Check sheet for the modelled part. Datum: model origin and axes. Units: mm. A direction names the side the tool comes from. Give positions to 0.01 mm unless a question says otherwise; leave off trailing zeros. Write each loop counter-clockwise with the first axis right and the second up, starting at its lowest first coordinate (ties: lowest second). Pieces come first, ordered by that corner, then holes. Notation, with made-up numbers: M -21.75,-32 L 26.25,-32 A22 cw 26.25,-25 Z; hole C 78.5,53 d10. An arc over 180 degrees is marked long. Write item = value, one per line. Start each with the question number.
1) Cross-section at A-A, the plane x = 13. Record the cut outline in (y, z) (3 decimals).
2) Access from +Z, -Z, +X, -X, +Y, -Y to the whole of each face (thin tool, end or side, straight path). Record for faces 4 (the cylindrical face through (0.456, 50.245, 136.744)), 5 (the flat face through (0, 25, 0)).
3) Mould release check, pull along Z, two halves, no side actions. Record for faces 1 (the cylindrical face through (0.46, 50.21, 23.34)), 2 (the flat face through (0, 25, 152.4)), 3 (the flat face through (-14.989, 19, 75)): released by +Z, released by -Z, zero draft, split by the parting line, or undercut.
4) Go/stop test with a flat-tipped pin: pin 1 (8 mm diameter, centred on x = -8, z = 66.5, fed in from +Y). Record where the tip stops, or that it passes through.
5) Scan lines: line 1 along Y through (x, z) = (1.5, 79.5); line 2 along Y through (x, z) = (14, 101); line 3 along Z through (x, y) = (-9.5, 48). Record each from-to range of solid material in increasing order. Write a range as [from, to].
```python
from build123d import *

# Parameters (mm, degrees)
F0_W     = 30.48
F0_H     = 152.4
F1_DEPTH = 50.8
F3_DEPTH = 30.481
F4_R     = 5.08


with BuildPart() as f1:
    # F0 (on Front) → F1 (new body)
    with BuildSketch(Plane.XZ):
        with Locations((0.2509840885, 76.2)):
            Rectangle(F0_W, F0_H)
    extrude(amount=-F1_DEPTH)

    # F2 (on face) → F3 (cut, through all)
    with BuildSketch(Plane.YZ.offset(15.4909840885)):
        with BuildLine():
            ThreePointArc((65.3252072253, 107.95), (71.4179823352, 113.7862789789), (73.66, 121.92))
            ThreePointArc((73.66, 121.92), (49.6512789789, 135.5529823352), (50.2447927747, 107.95))
            ThreePointArc((50.2447927747, 107.95), (57.785, 109.855), (65.3252072253, 107.95))
        make_face()
        with BuildLine():
            ThreePointArc((65.3252072253, 107.95), (57.785, 109.855), (50.2447927747, 107.95))
            ThreePointArc((50.2447927747, 107.95), (57.785, 106.045), (65.3252072253, 107.95))
        make_face()
        with BuildLine():
            ThreePointArc((65.3252072253, 107.95), (57.785, 106.045), (50.2447927747, 107.95))
            ThreePointArc((50.2447927747, 107.95), (41.91, 93.98), (50.2447927747, 80.01))
            ThreePointArc((50.2447927747, 80.01), (57.785, 81.915), (65.3252072253, 80.01))
            ThreePointArc((65.3252072253, 80.01), (71.4179823352, 85.8462789789), (73.66, 93.98))
            ThreePointArc((73.66, 93.98), (71.4179823352, 102.1137210211), (65.3252072253, 107.95))
        make_face()
        with BuildLine():
            ThreePointArc((65.3252072253, 80.01), (57.785, 81.915), (50.2447927747, 80.01))
            ThreePointArc((50.2447927747, 80.01), (57.785, 78.105), (65.3252072253, 80.01))
        make_face()
        with BuildLine():
            ThreePointArc((65.3252072253, 80.01), (57.785, 78.105), (50.2447927747, 80.01))
            ThreePointArc((50.2447927747, 80.01), (41.91, 66.04), (50.2447927747, 52.07))
            ThreePointArc((50.2447927747, 52.07), (57.785, 53.975), (65.3252072253, 52.07))
            ThreePointArc((65.3252072253, 52.07), (71.4179823352, 57.9062789789), (73.66, 66.04))
            ThreePointArc((73.66, 66.04), (71.4179823352, 74.1737210211), (65.3252072253, 80.01))
        make_face()
        with BuildLine():
            ThreePointArc((65.3252072253, 52.07), (57.785, 53.975), (50.2447927747, 52.07))
            ThreePointArc((50.2447927747, 52.07), (57.785, 50.165), (65.3252072253, 52.07))
        make_face()
        with BuildLine():
            ThreePointArc((65.3252072253, 52.07), (57.785, 50.165), (50.2447927747, 52.07))
            ThreePointArc((50.2447927747, 52.07), (49.6512789789, 24.4670176648), (73.66, 38.1))
            ThreePointArc((73.66, 38.1), (71.4179823352, 46.2337210211), (65.3252072253, 52.07))
        make_face()
    extrude(amount=-F3_DEPTH, mode=Mode.SUBTRACT)

    # F4
    f4_edges = [f1.edges().sort_by_distance(p)[0] for p in [
        (15.490984, 41.91307, 122.232205),
        (15.490984, 41.91307, 37.787795),
        (-14.989016, 41.91307, 122.232205),
        (-14.989016, 41.91, 93.98),
        (-14.989016, 41.91, 66.04),
        (-14.989016, 41.91307, 37.787795),
        (0.250984, 50.8, 23.844285),
        (0.250984, 50.8, 136.175715),
        (0.250984, 50.244793, 52.07),
        (15.490984, 41.91, 66.04),
        (0.250984, 50.244793, 80.01),
        (15.490984, 41.91, 93.98),
        (0.250984, 50.244793, 107.95),
    ]]
    fillet(f4_edges, radius=F4_R)


solid = f1.part
```
Reply:
q1.outline = M 0,0 L 50.8,0 L 50.8,20.967 A5.08 ccw 50.207,23.348 A16.584 cw 45.424,49.156 A4.371 ccw 45.424,54.984 A16.584 cw 45.424,77.096 A4.371 ccw 45.424,82.924 A16.584 cw 45.424,105.036 A4.371 ccw 45.424,110.864 A16.584 cw 50.207,136.672 A5.08 ccw 50.8,139.053 L 50.8,152.4 L 0,152.4 Z
q2.face_4 = +X, -X, +Y
q2.face_5 = -Z, +X, -X, +Y, -Y
q3.face_1 = undercut
q3.face_2 = released by +Z
q3.face_3 = zero draft
q4.pin_1 = 42.55
q5.line_1 = [0, 47.22]
q5.line_2 = [0, 41.91]
q5.line_3 = [0, 25.6], [134.42, 152.4]
